Work out the finished part from the listing and answer in its coordinate system (mm). A direction names the side the tool comes from. Round coordinates to 2 decimals unless told otherwise and drop trailing zeros. Loops run counter-clockwise (first coordinate to the right, second up) from the corner with the lowest first, then second, coordinate; pieces in that order, holes last.
Autodesk Inventor part; units mm, degrees
ref_plane "YZ Plane" through (0, 0, 0) normal (1, 0, 0) x (0, 1, 0)
ref_plane "XZ Plane" through (0, 0, 0) normal (0, 1, 0) x (-1, 0, 0)
ref_plane "XY Plane" through (0, 0, 0) normal (0, 0, 1) x (1, 0, 0)
sketch "Boceto1" plane through (0, 0, 0) normal (0, 1, 0) x (-1, 0, 0)
  line L0 (0, 0) -> (-6.7, 0)
  line L1 (-6.7, 0) -> (-6.7, -27.4)
  line L2 (-6.7, -27.4) -> (0, -27.4)
  line L3 (0, -27.4) -> (0, 0)
  line L4 (-7.7, 3) -> (1, 3)
  line L5 (3, 1) -> (3, -28.4)
  line L6 (1, -30.4) -> (-7.7, -30.4)
  line L7 (-9.7, -28.4) -> (-9.7, 1)
  arc A0 (3, 1) -> (1, 3) centre (1, 1) ccw
  arc A1 (-7.7, 3) -> (-9.7, 1) centre (-7.7, 1) ccw
  arc A2 (-9.7, -28.4) -> (-7.7, -30.4) centre (-7.7, -28.4) ccw
  arc A3 (1, -30.4) -> (3, -28.4) centre (1, -28.4) ccw
  dimension "d0" = 6.7
  dimension "d1" = 27.4
  dimension "d2" = 3
  dimension "d3" = 2
extrude "Extrusión1" add sketch "Boceto1" along normal blind 31
sketch "Boceto2" plane through (0, 0, 0) normal (0, -1, 0) x (1, 0, 0)
  line L0 (9.7, 1) -> (9.7, -28.4)
  arc A0 (9.7, 1) -> (7.7, 3) centre (7.7, 1) ccw
  line L1 (-1, 3) -> (7.7, 3)
  arc A1 (-1, 3) -> (-3, 1) centre (-1, 1) ccw
  line L2 (-3, -28.4) -> (-3, 1)
  arc A2 (-3, -28.4) -> (-1, -30.4) centre (-1, -28.4) ccw
  line L3 (7.7, -30.4) -> (-1, -30.4)
  arc A3 (7.7, -30.4) -> (9.7, -28.4) centre (7.7, -28.4) ccw
  point P0 (0, 0)
extrude "Extrusión2" add sketch "Boceto2" along normal blind 3
sketch "Boceto3" plane through (9.7, 31, 1) normal (1, 0, 0) x (0, 0, -1)
  line L0 (29.4, -34) -> (29.4, 0)
  line L1 (0, 0) -> (29.4, 0)
  line L2 (0, -34) -> (0, 0)
  line L3 (29.4, -34) -> (0, -34)
  line L4 (28.4, -31) -> (28.4, 0)
  line L5 (1, -31) -> (1, 0)
  line L6 (28.4, -31) -> (1, -31)
  line L7 (6, 0) -> (6, -26)
  line L8 (6, -26) -> (23.4, -26)
  line L9 (23.4, -26) -> (23.4, 0)
  line L10 (23.4, -26) -> (23.4, -31)
  line L11 (6, -26) -> (6, -31)
  point P0 (6, 0)
  dimension "d8" = 5
extrude "Extrusión3" cut sketch "Boceto3" against normal blind 3 contours L4 L6 L10 L9 L1 | L1 L7 L11 L6 L5
sketch "Boceto4" plane through (0, -3, 0) normal (0, -1, 0) x (1, 0, 0)
  line L0 (-3, 1) -> (-3, -28.4)
  line L1 (-3, -3.7) -> (-6.1, -3.7)
  line L2 (-6.1, -3.7) -> (-6.1, -0.6)
  line L3 (-6.1, -0.6) -> (-9.1, -0.6)
  line L4 (-3, -23.7) -> (-6.1, -23.7)
  line L5 (-6.1, -23.7) -> (-6.1, -26.8)
  line L6 (-6.1, -26.8) -> (-9.1, -26.8)
  line L7 (-9.1, -26.8) -> (-9.1, -0.6)
  line L8 (0, 0) -> (0, -27.4)
  point P0 (0, -13.7)
  dimension "d11" = 3.1
  dimension "d12" = 3.1
  dimension "d13" = 3
  dimension "d14" = 3.1
  dimension "d15" = 10
  dimension "d16" = 10
  dimension "d17" = 3.1
extrude "Extrusión4" add sketch "Boceto4" against normal up to surface (34 mm away)
sketch "Boceto5" plane through (0, -3, 0) normal (0, -1, 0) x (1, 0, 0)
  line L0 (9.7, 0) -> (0, 0)
  line L1 (9.7, -5) -> (9.7, 0)
  line L2 (9.7, -5) -> (6.7, -5)
  line L3 (6.7, -22.4) -> (6.7, -5)
  line L4 (9.7, -22.4) -> (6.7, -22.4)
  line L5 (9.7, -27.4) -> (9.7, -22.4)
  line L6 (0, -27.4) -> (9.7, -27.4)
  line L7 (0, 0) -> (0, -27.4)
  point P0 (2.5, -2.5)
  point P1 (2.5, -24.9)
  dimension "d20" = 2.5
  dimension "d21" = 2.5
hole "Agujero1" at (2.5, -3, -2.5) at (2.5, -3, -24.9) direction (0, 1, 0) diameter 4.5 end through all
properties part number "cajaEsp32Cam"
Item 1: Section C-C, the plane z = -24.9 is taken. Give the vertices of the cut face in (x, y), plus the area to 3 significant figures.
Item 2: Straight lines are drawn through the part: line 1 (Z direction, x = 2.5, y = -1.75); line 2 (Z direction, x = 6.75, y = 25.5); line 3 (X direction, y = 26, z = -7). For each, find the intervals that lie inside material, in ascending order.
Item 3: For faces 1 (the face through (-8, 14, -0.6)), 2 (the face through (-8, 14, -26.8)), 3 (the face through (-3, 14, -26)), determine the directions among +Z, -Z, +X, -X, +Y, -Y from which every point of the face is accessible in a straight line to the end or side of a thin tool.
Item 4: Each of these flat-tipped pins is pushed along its axis until it touches: P1, Ø0.9, axis at y = 21, z = -25, coming from the +X side; P2, Ø3.5, axis at x = -8, y = 14.5, coming from the +Z side; P3, Ø3.5, axis at y = 12.5, z = -1.5, coming from the +X side; P4, Ø3.5, axis at x = -4.5, y = 7, coming from the +Z side. Where does it stop, or does it pass through?
Item 5: Section D-D, the plane z = -10.5 is taken. Give the vertices of the cut face in (x, y).
Item 6: Determine the mould class of faces 4 (the face through (-2.43, 13.76, -29.8)), 5 (the face through (5, 15, 0)), 6 (the face through (8, 16, -5)), 7 (the face through (-6.1, 14, -2)) for opening direction Z: pulls with the +Z half, pulls with the -Z half, needs draft (parallel to the pull), parting line crosses it, or undercut.
Item 7: Section B-B, the plane x = 2.5 is taken. Give the vertices of the cut face in (y, z), plus the area to 3 significant figures.
Item 8: Section A-A, the plane y = 22 is taken. Give the vertices of the cut face in (x, z), plus the area to 3 significant figures.
Answer below:
1. outline: (-9.1, -3) - (-6.1, -3) - (-6.1, 31) - (-9.1, 31) - close; (-3, -3) - (0.25, -3) - (0.25, 0) - (0, 0) - (0, 31) - (-3, 31) - close; (4.75, -3) - (9.7, -3) - (9.7, 0) - (4.75, 0) - close
1. area: 220 mm2
2. line 1: z = -30.4 to -27.15, -22.65 to -4.75, -0.25 to 3
2. line 2: z = -30.4 to -27.4, -22.4 to -5, 0 to 3
2. line 3: x = -9.1 to 0, 6.7 to 9.7
3. face 1: +Z, -X, +Y, -Y
3. face 2: -Z, -X, +Y, -Y
3. face 3: -Z, +Y, -Y
4. P1: stops at x = 0
4. P2: stops at z = -0.6
4. P3: stops at x = 9.7
4. P4: stops at z = 1.97
5. outline: (-9.1, -3) - (9.7, -3) - (9.7, 31) - (6.7, 31) - (6.7, 0) - (0, 0) - (0, 31) - (-9.1, 31) - close
6. face 4: pulls with the -Z half
6. face 5: undercut
6. face 6: undercut
6. face 7: needs draft
7. outline: (-3, -30.4) - (31, -30.4) - (31, -27.4) - (0, -27.4) - (0, -27.15) - (-3, -27.15) - close; (-3, -22.65) - (0, -22.65) - (0, -4.75) - (-3, -4.75) - close; (-3, -0.25) - (0, -0.25) - (0, 0) - (31, 0) - (31, 3) - (-3, 3) - close
7. area: 259 mm2
8. outline: (-9.1, -26.8) - (-6.1, -26.8) - (-6.1, -23.7) - (-3, -23.7) - (-3, -28.4) arc R2 ccw to (-1, -30.4) - (7.7, -30.4) arc R2 ccw to (9.7, -28.4) - (9.7, -27.4) - (0, -27.4) - (0, 0) - (9.7, 0) - (9.7, 1) arc R2 ccw to (7.7, 3) - (-1, 3) arc R2 ccw to (-3, 1) - (-3, -3.7) - (-6.1, -3.7) - (-6.1, -0.6) - (-9.1, -0.6) - close; (6.7, -22.4) - (9.7, -22.4) - (9.7, -5) - (6.7, -5) - close
8. area: 348 mm2
